Source: CAD feature listing. Evaluate the final solid. Frame: model axes, mm. Coordinates: 2 decimals unless noted, no trailing zeros. Order: outer loops, then holes, each group sorted by start corner. A loop starts at its lowest first (then second) coordinate and runs counter-clockwise, first axis right, second up. Notation, with made-up numbers: (63, 19.5) -> (67, 19.5) arc R36 cw to (67, 53.5) -> close; hole circle Ø3 at (-36, -26.75). An arc over 180 degrees is marked (long way). Put each result on its own line as item: value.
from build123d import *

# Parameters (mm, degrees)
GE_24334_OUTLINE_R   = 5.3578125
GE_24334_OUTLINE_R_2 = 3.373501
GE_24334_DEPTH       = 6.35
SKETCH1_W            = 1036.405519013
SKETCH1_H            = 5.842
CUT_EXTRUDE1_DEPTH   = 1400.059095494


# Read off the part's stored shape, not the designer's step: GE-24334
with BuildPart() as part:
    # GE-24334 outline → GE-24334 (new body)
    with BuildSketch(Plane.XY):
        with BuildLine():
            ThreePointArc((133.104268735, 292.971606529), (129.401623275, 291.780377371), (127.088174424, 288.653627505))
            Line((127.088174424, 288.653627505), (-262.322220882, -864.25261299))
            ThreePointArc((-262.322220882, -864.25261299), (-261.464897413, -869.987279425), (-256.306126571, -872.634633965))
            Line((-256.306126571, -872.634633965), (767.399392442, -872.634633965))
            ThreePointArc((767.399392442, -872.634633965), (772.558163284, -869.987279425), (773.415486753, -864.25261299))
            Line((773.415486753, -864.25261299), (384.005091446, 288.653627505))
            ThreePointArc((384.005091446, 288.653627505), (381.691642596, 291.780377371), (377.988997136, 292.971606529))
            Line((377.988997136, 292.971606529), (133.104268735, 292.971606529))
        make_face()
        with BuildLine():
            Line((-180.239726648, -736.327985402), (-172.111642745, -712.26360816))
            ThreePointArc((-172.111642745, -712.26360816), (-156.015412172, -704.29546149), (-148.047265502, -720.391692063))
            Line((-148.047265502, -720.391692063), (-156.175349405, -744.456069305))
            ThreePointArc((-156.175349405, -744.456069305), (-172.271579978, -752.424215975), (-180.239726648, -736.327985402))
        make_face(mode=Mode.SUBTRACT)
        with Locations((-82.126785136, -834.534633965)):
            Circle(GE_24334_OUTLINE_R, mode=Mode.SUBTRACT)
        with BuildLine():
            Line((-94.231734473, -791.354633965), (-68.831734473, -791.354633965))
            ThreePointArc((-68.831734473, -791.354633965), (-56.131734473, -804.054633965), (-68.831734473, -816.754633965))
            Line((-68.831734473, -816.754633965), (-94.231734473, -816.754633965))
            ThreePointArc((-94.231734473, -816.754633965), (-106.931734473, -804.054633965), (-94.231734473, -791.354633965))
        make_face(mode=Mode.SUBTRACT)
        with Locations((-81.003367065, -777.384633965)):
            Circle(GE_24334_OUTLINE_R_2, mode=Mode.SUBTRACT)
        with Locations((-193.570796303, -720.234633965)):
            Circle(GE_24334_OUTLINE_R, mode=Mode.SUBTRACT)
        with Locations((-82.126785136, -390.288393471)):
            Circle(GE_24334_OUTLINE_R, mode=Mode.SUBTRACT)
        with BuildLine():
            Line((-68.772097635, -406.311820835), (-60.644013732, -382.247443592))
            ThreePointArc((-60.644013732, -382.247443592), (-44.54778316, -374.279296923), (-36.57963649, -390.375527495))
            Line((-36.57963649, -390.375527495), (-44.707720392, -414.439904738))
            ThreePointArc((-44.707720392, -414.439904738), (-60.803950965, -422.408051408), (-68.772097635, -406.311820835))
        make_face(mode=Mode.SUBTRACT)
        with Locations((593.220051006, -834.534633965)):
            Circle(GE_24334_OUTLINE_R, mode=Mode.SUBTRACT)
        with BuildLine():
            Line((580.520051006, -791.354633965), (605.920051006, -791.354633965))
            ThreePointArc((605.920051006, -791.354633965), (618.620051006, -804.054633965), (605.920051006, -816.754633965))
            Line((605.920051006, -816.754633965), (580.520051006, -816.754633965))
            ThreePointArc((580.520051006, -816.754633965), (567.820051006, -804.054633965), (580.520051006, -791.354633965))
        make_face(mode=Mode.SUBTRACT)
        with Locations((592.096632935, -777.384633965)):
            Circle(GE_24334_OUTLINE_R_2, mode=Mode.SUBTRACT)
        with BuildLine():
            Line((667.268615276, -744.456069305), (659.140531373, -720.391692063))
            ThreePointArc((659.140531373, -720.391692063), (667.108678043, -704.29546149), (683.204908616, -712.26360816))
            Line((683.204908616, -712.26360816), (691.332992518, -736.327985402))
            ThreePointArc((691.332992518, -736.327985402), (683.364845849, -752.424215975), (667.268615276, -744.456069305))
        make_face(mode=Mode.SUBTRACT)
        with Locations((704.664062174, -720.234633965)):
            Circle(GE_24334_OUTLINE_R, mode=Mode.SUBTRACT)
        with BuildLine():
            Line((555.800986263, -414.439904738), (547.67290236, -390.375527495))
            ThreePointArc((547.67290236, -390.375527495), (555.64104903, -374.279296923), (571.737279603, -382.247443592))
            Line((571.737279603, -382.247443592), (579.865363506, -406.311820835))
            ThreePointArc((579.865363506, -406.311820835), (571.897216836, -422.408051408), (555.800986263, -414.439904738))
        make_face(mode=Mode.SUBTRACT)
        with Locations((593.220051006, -390.288393471)):
            Circle(GE_24334_OUTLINE_R, mode=Mode.SUBTRACT)
        with Locations((-23.853367065, -269.384633965)):
            Circle(GE_24334_OUTLINE_R_2, mode=Mode.SUBTRACT)
        with Locations((19.96580657, -88.028393471)):
            Circle(GE_24334_OUTLINE_R, mode=Mode.SUBTRACT)
        with BuildLine():
            Line((33.202373314, -104.401534553), (41.330457217, -80.33715731))
            ThreePointArc((41.330457217, -80.33715731), (57.42668779, -72.36901064), (65.394834459, -88.465241213))
            Line((65.394834459, -88.465241213), (57.266750557, -112.529618456))
            ThreePointArc((57.266750557, -112.529618456), (41.170519984, -120.497765125), (33.202373314, -104.401534553))
        make_face(mode=Mode.SUBTRACT)
        with Locations((114.659199441, 192.325199783)):
            Circle(GE_24334_OUTLINE_R, mode=Mode.SUBTRACT)
        with BuildLine():
            Line((127.949253412, 176.110415433), (136.077337315, 200.174792676))
            ThreePointArc((136.077337315, 200.174792676), (152.173567887, 208.142939345), (160.141714557, 192.046708773))
            Line((160.141714557, 192.046708773), (152.013630654, 167.98233153))
            ThreePointArc((152.013630654, 167.98233153), (135.917400081, 160.01418486), (127.949253412, 176.110415433))
        make_face(mode=Mode.SUBTRACT)
        with BuildLine():
            Line((192.113515822, 253.947158802), (217.513515822, 253.947158802))
            ThreePointArc((217.513515822, 253.947158802), (230.213515822, 241.247158802), (217.513515822, 228.547158802))
            Line((217.513515822, 228.547158802), (192.113515822, 228.547158802))
            ThreePointArc((192.113515822, 228.547158802), (179.413515822, 241.247158802), (192.113515822, 253.947158802))
        make_face(mode=Mode.SUBTRACT)
        with Locations((204.746632935, 271.727158802)):
            Circle(GE_24334_OUTLINE_R, mode=Mode.SUBTRACT)
        with BuildLine():
            Line((453.826515314, -112.529618456), (445.698431411, -88.465241213))
            ThreePointArc((445.698431411, -88.465241213), (453.666578081, -72.36901064), (469.762808654, -80.33715731))
            Line((469.762808654, -80.33715731), (477.890892557, -104.401534553))
            ThreePointArc((477.890892557, -104.401534553), (469.922745887, -120.497765125), (453.826515314, -112.529618456))
        make_face(mode=Mode.SUBTRACT)
        with Locations((491.127459301, -88.028393471)):
            Circle(GE_24334_OUTLINE_R, mode=Mode.SUBTRACT)
        with Locations((534.946632935, -269.384633965)):
            Circle(GE_24334_OUTLINE_R_2, mode=Mode.SUBTRACT)
        with BuildLine():
            Line((359.065010443, 168.025630302), (350.936926541, 192.090007545))
            ThreePointArc((350.936926541, 192.090007545), (358.90507321, 208.186238118), (375.001303783, 200.218091448))
            Line((375.001303783, 200.218091448), (383.129387686, 176.153714205))
            ThreePointArc((383.129387686, 176.153714205), (375.161241016, 160.057483633), (359.065010443, 168.025630302))
        make_face(mode=Mode.SUBTRACT)
        with BuildLine():
            Line((293.646632935, 253.947158802), (319.046632935, 253.947158802))
            ThreePointArc((319.046632935, 253.947158802), (331.746632935, 241.247158802), (319.046632935, 228.547158802))
            Line((319.046632935, 228.547158802), (293.646632935, 228.547158802))
            ThreePointArc((293.646632935, 228.547158802), (280.946632935, 241.247158802), (293.646632935, 253.947158802))
        make_face(mode=Mode.SUBTRACT)
        with Locations((306.346632935, 271.727158802)):
            Circle(GE_24334_OUTLINE_R, mode=Mode.SUBTRACT)
        with Locations((396.756156044, 191.371606529)):
            Circle(GE_24334_OUTLINE_R, mode=Mode.SUBTRACT)
    extrude(amount=GE_24334_DEPTH)

    # Sketch1 → Cut-Extrude1 (cut, through all)
    with BuildSketch(Plane.XZ.offset(872.634633965)):
        with Locations((255.546632936, 3.429)):
            Rectangle(SKETCH1_W, SKETCH1_H)
    extrude(amount=-CUT_EXTRUDE1_DEPTH, mode=Mode.SUBTRACT)


solid = part.part
1. Cut plane C-C on x = 429. Output: boundary loops of the cut face in (y, z).
Numbers:
outline: (-872.63, 0) -> (155.44, 0) -> (155.44, 0.51) -> (-872.63, 0.51) -> close
2. Cut plane A-A on z = 0.2. Count the separate pieces of the cut face and the enclosed holes in it, plus the area to 3 significant figures.
Numbers:
separate pieces: 1
enclosed holes: 28
area: 740,000 mm2
3. Ray query, line 1 along Y through (x, z) = (146, 0.2); line 2 along X through (y, z) = (-779.5, 0.3); line 3 along X through (y, z) = (-141, 0.2). Return the intervals inside material, ascending.
Numbers:
line 1: y = -872.63 to 160.86, 208.63 to 292.97
line 2: x = -233.7 to -83.63, -78.38 to 589.47, 594.72 to 744.79
line 3: x = -18.03 to 529.13
4. Cut plane B-B on y = -311.5. Output: boundary loops of the cut face in (x, z), plus the area to 3 significant figures.
Numbers:
outline: (-75.62, 0) -> (586.72, 0) -> (586.72, 0.51) -> (-75.62, 0.51) -> close
area: 336 mm2
